The figure shows three views and two pictorial views of one solid part (mm, origin at its lowest corner). Answer the questions. Give positions to 0.01 mm unless a question says otherwise; leave off trailing zeros. Loops run counter-clockwise (first coordinate to the right, second up) from the corner with the lowest first, then second, coordinate; pieces in that order, holes last. Notation, with made-up numbers: (-5.75, 59) - (18.25, 59) arc R22 ccw to (18.25, 91) - close; hole circle Ø10 at (54, 14). An arc over 180 degrees is marked (long way). Use a Markdown table: item, result. Add a question column.
Item 1: A cutting plane is placed at A-A (z = 30). Determine the outline of the cut face in (x, y), plus the area to 3 significant figures.
Item 2: A cutting plane is placed at C-C (y = 2.75). Determine the outline of the cut face in (x, z), plus the area to 3 significant figures.
Item 3: For a pull along X with two mould halves and no side action, classify the marked faces 1, 2 and 3 as +X half, -X half, draft (parallel to the pull), parting line (faces both ways), or undercut.
Item 4: Consider probe 1 along Z at (x, y) = (30, 11); probe 2 along Y at (x, z) = (5, 17); probe 3 along X at (y, z) = (20, 13). Determine where each line is inside the solid, lowest interval first. Write a range as [from, to].
Item 5: A cutting plane is placed at D-D (z = 8.5). Determine the outline of the cut face in (x, y), plus the area to 3 significant figures.
Item 6: Each of these flat-tipped pins is pushed along its axis until it touches: P1, Ø6, axis at y = 3.5, z = 42.5, coming from the +X side; P2, Ø10, axis at x = 29.5, y = 13, coming from the +Z side; P3, Ø1, axis at y = 9.5, z = 36.5, coming from the +X side. Where does it stop, or does it pass through?
Item 7: A cutting plane is placed at B-B (x = 30). Determine the outline of the cut face in (y, z).
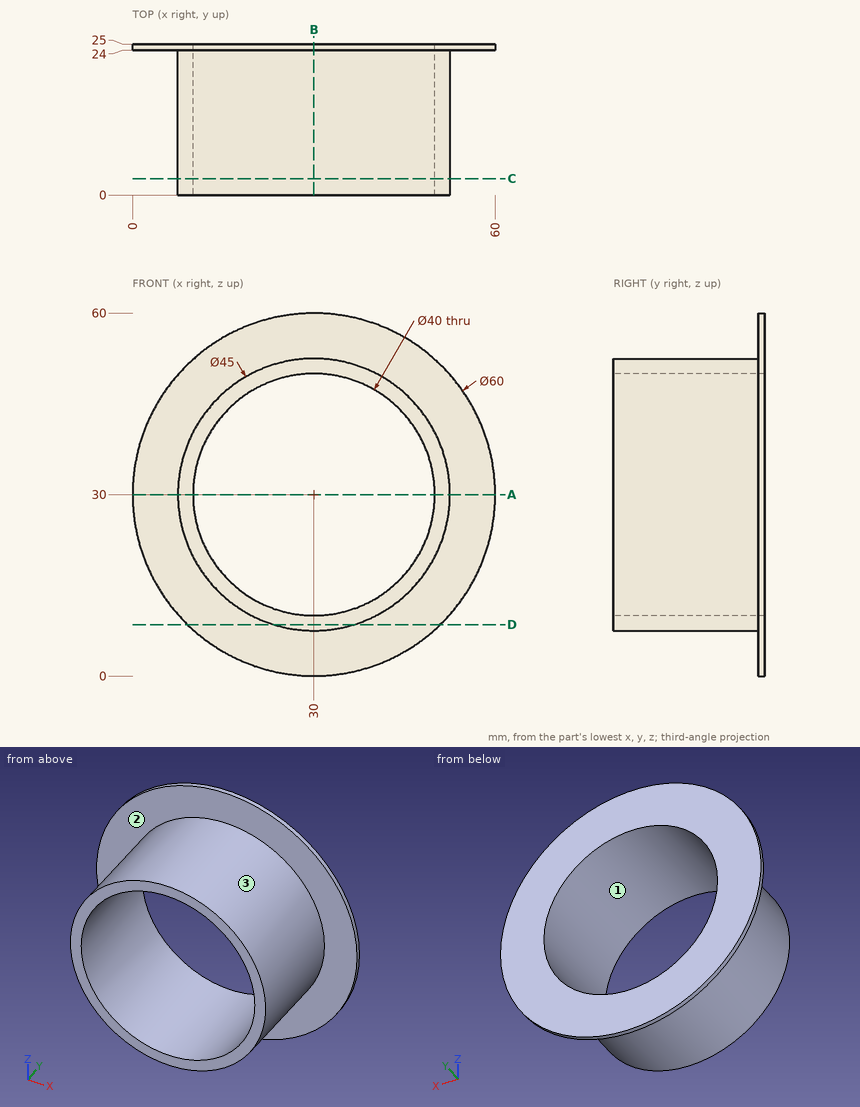
Geometry says:
| question | item | result |
|---|---|---|
| 1 | outline | (0, 24) - (7.5, 24) - (7.5, 0) - (10, 0) - (10, 25) - (0, 25) - close; (50, 0) - (52.5, 0) - (52.5, 24) - (60, 24) - (60, 25) - (50, 25) - close |
| 1 | area | 140 mm² |
| 2 | outline | circle Ø45 at (30, 30); hole circle Ø40 at (30, 30) |
| 2 | area | 334 mm² |
| 3 | face 1 | undercut |
| 3 | face 2 | draft |
| 3 | face 3 | parting line |
| 4 | probe 1 | [7.5, 10], [50, 52.5] |
| 4 | probe 2 | [24, 25] |
| 4 | probe 3 | [15.26, 19.46], [40.54, 44.74] |
| 5 | outline | (9.08, 24) - (23.37, 24) - (23.37, 0) - (36.63, 0) - (36.63, 24) - (50.92, 24) - (50.92, 25) - (9.08, 25) - close |
| 5 | area | 360 mm² |
| 6 | P1 | x = 50.4 |
| 6 | P2 | z = 52.5 |
| 6 | P3 | x = 51.69 |
| 7 | outline | (0, 7.5) - (24, 7.5) - (24, 0) - (25, 0) - (25, 10) - (0, 10) - close; (0, 50) - (25, 50) - (25, 60) - (24, 60) - (24, 52.5) - (0, 52.5) - close |
